Here's how the part is built. I have some questions about the finished solid (model axes, mm). Coordinates: 2 decimals unless noted, no trailing zeros. Write each loop counter-clockwise with the first axis right and the second up, starting at its lowest first coordinate (ties: lowest second). Pieces come first, ordered by that corner, then holes.
```python
from build123d import *

# Parameters (mm, degrees)
BOSS_EXTRUDE1_START                             = -32.7
SKETCH2_R                                       = 3
BOSS_EXTRUDE1_DEPTH                             = 4
FILLET1_R                                       = 6
CSK_FOR_M3_FLAT_HEAD_MACHINE_SCREW1_D           = 3.6
CSK_FOR_M3_FLAT_HEAD_MACHINE_SCREW1_CSINK_D     = 6.3
CSK_FOR_M3_FLAT_HEAD_MACHINE_SCREW1_CSINK_ANGLE = 90


with BuildPart() as part:
    # Sketch2 → Boss-Extrude1 (new body)
    # profile 1 of 4: a face of its own
    with BuildSketch(Plane(origin=(0, 0, 0), x_dir=(0, 0, -1), z_dir=(1, 0, 0)).offset(BOSS_EXTRUDE1_START)):
        with BuildLine():
            Line((26, -4.467659364), (26, -30.118056984))
            ThreePointArc((26, -30.118056984), (0, -16), (-26, -30.118056984))
            Line((-26, -30.118056984), (-26, -4.467659364))
            ThreePointArc((-26, -4.467659364), (-25.065528054, -1.252006159), (-22.553191489, 0.962001143))
            ThreePointArc((-22.553191489, 0.962001143), (0, 6), (22.553191489, 0.962001143))
            ThreePointArc((22.553191489, 0.962001143), (25.065528054, -1.252006159), (26, -4.467659364))
        make_face()
        with Locations((15, -2.457885097)):
            Circle(SKETCH2_R, mode=Mode.SUBTRACT)
        Circle(SKETCH2_R, mode=Mode.SUBTRACT)
        with Locations((-15, -2.457885097)):
            Circle(SKETCH2_R, mode=Mode.SUBTRACT)
    # profile 2 of 4: a face of its own
    with BuildSketch(Plane(origin=(0, 0, 0), x_dir=(0, 0, -1), z_dir=(1, 0, 0)).offset(BOSS_EXTRUDE1_START)):
        with Locations((-15, -2.457885097)):
            Circle(SKETCH2_R)
    # profile 3 of 4: a face of its own
    with BuildSketch(Plane(origin=(0, 0, 0), x_dir=(0, 0, -1), z_dir=(1, 0, 0)).offset(BOSS_EXTRUDE1_START)):
        Circle(SKETCH2_R)
    # profile 4 of 4: a face of its own
    with BuildSketch(Plane(origin=(0, 0, 0), x_dir=(0, 0, -1), z_dir=(1, 0, 0)).offset(BOSS_EXTRUDE1_START)):
        with Locations((15, -2.457885097)):
            Circle(SKETCH2_R)
    extrude(amount=-BOSS_EXTRUDE1_DEPTH)

    # Fillet1
    fillet1_edges = [part.edges().sort_by_distance(p)[0] for p in [
        (-34.7, -30.118056984, -26),
        (-34.7, -30.118056984, 26),
    ]]
    fillet(fillet1_edges, radius=FILLET1_R)

    # CSK for M3 Flat Head Machine Screw1 (through all)
    with Locations(Plane(origin=(-32.7, 0, 0), x_dir=(0, 0, -1), z_dir=(1, 0, 0))):
        with Locations((-20, -4.467659364), (20, -4.467659364)):
            CounterSinkHole(CSK_FOR_M3_FLAT_HEAD_MACHINE_SCREW1_D / 2, CSK_FOR_M3_FLAT_HEAD_MACHINE_SCREW1_CSINK_D / 2, counter_sink_angle=CSK_FOR_M3_FLAT_HEAD_MACHINE_SCREW1_CSINK_ANGLE)


solid = part.part
```
1) Imagine slicing it at D-D on y = -20. Please give me the cut outline in (x, z).
Values follow:
outline: (-36.7, -24.35) - (-32.7, -24.35) - (-32.7, -15.23) - (-36.7, -15.23) - close; (-36.7, 15.23) - (-32.7, 15.23) - (-32.7, 24.35) - (-36.7, 24.35) - close
2) Imagine slicing it at B-B on y = -16.75. Please give me the cut outline in (x, z).
Values follow:
outline: (-36.7, -25.94) - (-32.7, -25.94) - (-32.7, -6.78) - (-36.7, -6.78) - close; (-36.7, 6.78) - (-32.7, 6.78) - (-32.7, 25.94) - (-36.7, 25.94) - close
3) Imagine slicing it at A-A on x = -34.6. Please give me the cut outline in (y, z).
Values follow:
outline: (-20.92, -16.76) arc R6 ccw to (-15.87, -26) - (-4.47, -26) arc R6 ccw to (0.96, -22.55) arc R53 ccw to (0.96, 22.55) arc R6 ccw to (-4.47, 26) - (-15.87, 26) arc R6 ccw to (-20.92, 16.76) arc R31 cw to start; hole circle Ø3.6 at (-4.47, -20); hole circle Ø3.6 at (-4.47, 20)
4) Will these pins go through, and if not, where does the flat tip stop? pin 1 (1.5 mm diameter, centred on x = -35, z = 3, fed in from +Y); pin 2 (4 mm diameter, centred on y = -4.47, z = 20, fed in from +X).
Values follow:
pin 1: stops at y = 5.95
pin 2: stops at x = -33.85
5) I need wall thicknesses on probe 1 along Y at (x, z) = (-34.8, 0.5); probe 2 along Y at (x, z) = (-33.6, 22); probe 3 along Z at (x, y) = (-34.4, -5.75). Which ranges of each line are inside material? Lowest first, please.
Values follow:
probe 1: y = -16 to 6
probe 2: y = -21.53 to -5.5, -3.44 to 1.22
probe 3: z = -26 to -21.26, -18.74 to 18.74, 21.26 to 26
6) We'd pull the mould along Z, two halves only. Please class faces 1 (the face through (-34.728, -21.093, -22.954)), 2 (the face through (-32.7, -8, 0)), 3 (the face through (-34.67, -1.21, -25.04)): pulls with the +Z half, pulls with the -Z half, needs draft (parallel to the pull), parting line crosses it, or undercut.
Values follow:
face 1: undercut
face 2: needs draft
face 3: pulls with the -Z half
7) Imagine slicing it at C-C on z = -20. Please give me the cut outline in (x, y).
Values follow:
outline: (-36.7, -21.87) - (-32.7, -21.87) - (-32.7, -7.62) - (-34.05, -6.27) - (-36.7, -6.27) - close; (-36.7, -2.67) - (-34.05, -2.67) - (-32.7, -1.32) - (-32.7, 2.08) - (-36.7, 2.08) - close
